from build123d import *

# Parameters (mm, degrees)
BOSS_EXTRUDE1_DEPTH = 10
FILLET1_R           = 4


with BuildPart() as part:
    # Sketch1 → Boss-Extrude1 (new body)
    with BuildSketch(Plane(origin=(0, 0, 0), x_dir=(1, 0, 0), z_dir=(0, 1, 0))):
        with BuildLine():
            Line((0, -10), (0, -28))
            Line((0, -28), (3, -28))
            Line((3, -28), (3, -9.539392014))
            ThreePointArc((3, -9.539392014), (6.47547653, -7.620249583), (8.93028555, -4.5))
            Line((8.93028555, -4.5), (14.367496998, -4.5))
            Line((14.367496998, -4.5), (14.367496998, -0.5))
            Line((14.367496998, -0.5), (9.987492178, -0.5))
            Line((9.987492178, -0.5), (7.984359711, -0.5))
            ThreePointArc((7.984359711, -0.5), (-8, 0), (7.984359711, 0.5))
            Line((7.984359711, 0.5), (9.987492178, 0.5))
            Line((9.987492178, 0.5), (14.367496998, 0.5))
            Line((14.367496998, 0.5), (14.367496998, 3.5))
            Line((14.367496998, 3.5), (9.367496998, 3.5))
            ThreePointArc((9.367496998, 3.5), (-8.215838363, 5.700877125), (0, -10))
        make_face()
    extrude(amount=BOSS_EXTRUDE1_DEPTH)

    # Fillet1
    fillet1_edges = [part.edges().sort_by_distance(p)[0] for p in [
        (8.93028555, 5, 4.5),
        (3, 5, 9.539392014),
        (0, 5, 10),
        (9.367496998, 5, -3.5),
    ]]
    fillet(fillet1_edges, radius=FILLET1_R)


solid = part.part
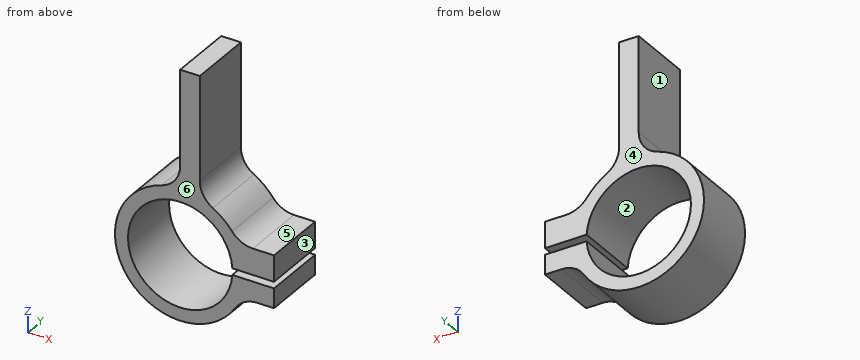
Work out the finished part from the listing and answer in its coordinate system (mm). Face numbers are marked on the shaded views. A direction names the side the tool comes from. Round coordinates to 2 decimals unless told otherwise and drop trailing zeros. Order: outer loops, then holes, each group sorted by start corner. A loop starts at its lowest first (then second) coordinate and runs counter-clockwise, first axis right, second up. Notation, with made-up numbers: M -32.5,16 L 21.5,16 A25 ccw 21.5,55 Z; hole C 79.5,48.5 d5. An arc over 180 degrees is marked long. Put each result on its own line as item: value. Start each with the question number.
Q1. A tool of negligible diameter and unlimited length cuts with its end or side. For the marked faces 5 and 6, from which of +Z, -Z, +X, -X, +Y, -Y can it reach the whole face along a straight path? Write none if from no direction.
Q2. Section B-B, the plane y = 5.5 is taken. Write down the section's boundary in (x, z).
Q3. Straight lines are drawn through the part: L1, parallel to Z at x = 12.5, y = 6.5; L2, parallel to X at y = 3, z = 14; L3, parallel to X at y = 3.25, z = 1.5. For each, find the intervals that lie inside material, in ascending order. Write a range as [from, to].
Q4. Flat-ended cylindrical pins translate along their axes: pin 1 (3 mm diameter, centred on y = 3, z = 18.5, fed in from -X); pin 2 (0.8 mm diameter, centred on x = 13, y = 5, fed in from -Z); pin 3 (3 mm diameter, centred on x = 12.5, y = 6, fed in from -Z); pin 4 (12 mm diameter, centred on x = 8.5, z = 12, fed in from +Y). Find the tip coordinate at first contact, or state that the pin passes through.
Q5. Section D-D, the plane z = 15 is taken. Write down the section's boundary in (x, y).
Q6. For a pull along X with two mould halves and no side action, classify the marked faces 1, 2, 3 and 4 as pulls with the +X half, pulls with the -X half, needs draft (parallel to the pull), parting line crosses it, or undercut.
Q7. Section A-A, the plane z = 1 is taken. Write down the section's boundary in (x, y), and give its area (3 significant figures).
Q8. Section C-C, the plane x = 7.5 is taken. Write down the section's boundary in (y, z).
Findings below:
1. face 5: +Z, +X, +Y, -Y
1. face 6: +Z, -Z, +X, -X, -Y
2. outline: M -2.86,9.58 A10 ccw long 8.44,-5.36 A4 cw 11.82,-3.5 L 14.37,-3.5 L 14.37,-0.5 L 7.98,-0.5 A8 cw long 7.98,0.5 L 14.37,0.5 L 14.37,4.5 L 11.12,4.5 A4 cw 7.95,6.07 A10 ccw 5,8.66 A4 cw 3,12.12 L 3,28 L 0,28 L 0,13.42 A4 cw Z
3. L1: z = [-3.5, -0.5], [0.5, 4.5]
3. L2: x = [0, 3]
3. L3: x = [-9.89, -7.86], [7.86, 14.37]
4. pin 1: stops at x = 0
4. pin 2: stops at z = -3.5
4. pin 3: stops at z = -3.59
4. pin 4: stops at y = 10
5. outline: M 0,0 L 3,0 L 3,10 L 0,10 Z
6. face 1: pulls with the -X half
6. face 2: undercut
6. face 3: pulls with the +X half
6. face 4: needs draft
7. outline: M -9.95,0 L -7.94,0 L -7.94,10 L -9.95,10 Z; M 7.94,0 L 14.37,0 L 14.37,10 L 7.94,10 Z
7. area: 84.4 mm^2
8. outline: M 0,-6.61 L 10,-6.61 L 10,-2.78 L 0,-2.78 Z; M 0,2.78 L 10,2.78 L 10,6.61 L 0,6.61 Z
